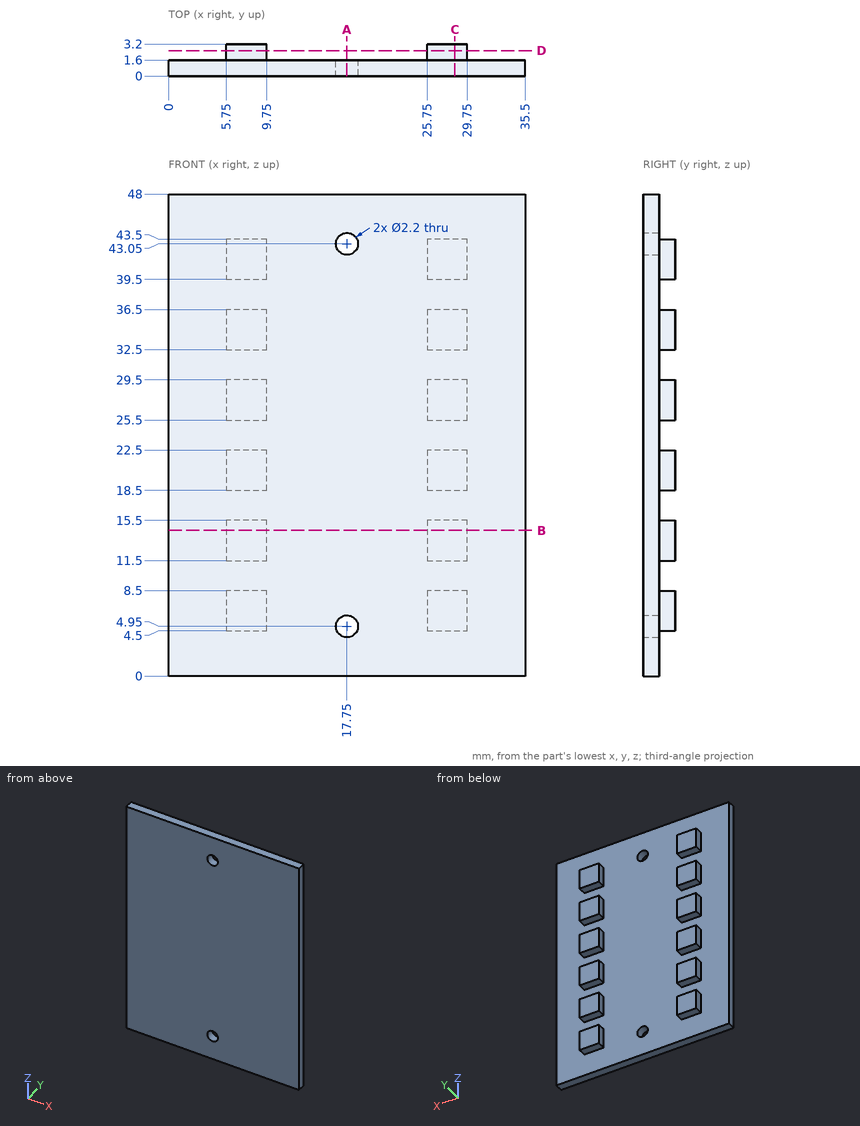
Answer from the drawing. Dimensions are ordinates in mm from the lowest x, y and z of the part. Give positions to 0.01 mm unless a question says otherwise; leave off trailing zeros. Write each loop counter-clockwise with the first axis right and the second up, starting at its lowest first coordinate (ties: lowest second). Pieces come first, ordered by that corner, then holes. Notation, with made-up numbers: (83, -9.75) -> (107, -9.75) arc R29 cw to (107, 15.25) -> close; hole circle Ø1 at (18, 11.5). An arc over 180 degrees is marked (long way). One line per question, with ' | ' between items. Start each with the question number.
1. Find the intervals of material crossed by probe 1 along Z at (x, y) = (17.75, 1); probe 2 along X at (y, z) = (0.4, 43.05); probe 3 along Z at (x, y) = (17, 1.4), in increasing order.
2. Section D-D (y = 2.55) is taken. State how many separate pieces and enclosed holes the cut face has, plus the area to 3 significant figures.
3. Given pin 1 Ø0.8 at (x, y) = (28, 2.5) entering from +Z; pin 2 Ø0.5 at (x, y) = (27, 2.5) entering from -Z; pin 3 Ø1.3 at (y, z) = (2.5, 35) entering from +X, each flat-ended and moving along its own axis, determine where each tip first touches the part or whether it passes through.
4. Section C-C (x = 28.5) is taken. Determine the outline of the cut face in (y, z), plus the area to 3 significant figures.
5. Section A-A (x = 17.75) is taken. Determine the outline of the cut face in (y, z).
6. Section B-B (z = 14.5) is taken. Determine the outline of the cut face in (x, y).
Response values:
1) probe 1: 0 to 3.85, 6.05 to 41.95, 44.15 to 48 | probe 2: 0 to 16.65, 18.85 to 35.5 | probe 3: 0 to 4.15, 5.75 to 42.25, 43.85 to 48
2) separate pieces: 12 | enclosed holes: 0 | area: 192 mm2
3) pin 1: z = 43.5 | pin 2: z = 4.5 | pin 3: x = 29.75
4) outline: (0, 0) -> (1.6, 0) -> (1.6, 4.5) -> (3.2, 4.5) -> (3.2, 8.5) -> (1.6, 8.5) -> (1.6, 11.5) -> (3.2, 11.5) -> (3.2, 15.5) -> (1.6, 15.5) -> (1.6, 18.5) -> (3.2, 18.5) -> (3.2, 22.5) -> (1.6, 22.5) -> (1.6, 25.5) -> (3.2, 25.5) -> (3.2, 29.5) -> (1.6, 29.5) -> (1.6, 32.5) -> (3.2, 32.5) -> (3.2, 36.5) -> (1.6, 36.5) -> (1.6, 39.5) -> (3.2, 39.5) -> (3.2, 43.5) -> (1.6, 43.5) -> (1.6, 48) -> (0, 48) -> close | area: 115 mm2
5) outline: (0, 0) -> (1.6, 0) -> (1.6, 3.85) -> (0, 3.85) -> close; (0, 6.05) -> (1.6, 6.05) -> (1.6, 41.95) -> (0, 41.95) -> close; (0, 44.15) -> (1.6, 44.15) -> (1.6, 48) -> (0, 48) -> close
6) outline: (0, 0) -> (35.5, 0) -> (35.5, 1.6) -> (29.75, 1.6) -> (29.75, 3.2) -> (25.75, 3.2) -> (25.75, 1.6) -> (9.75, 1.6) -> (9.75, 3.2) -> (5.75, 3.2) -> (5.75, 1.6) -> (0, 1.6) -> close
